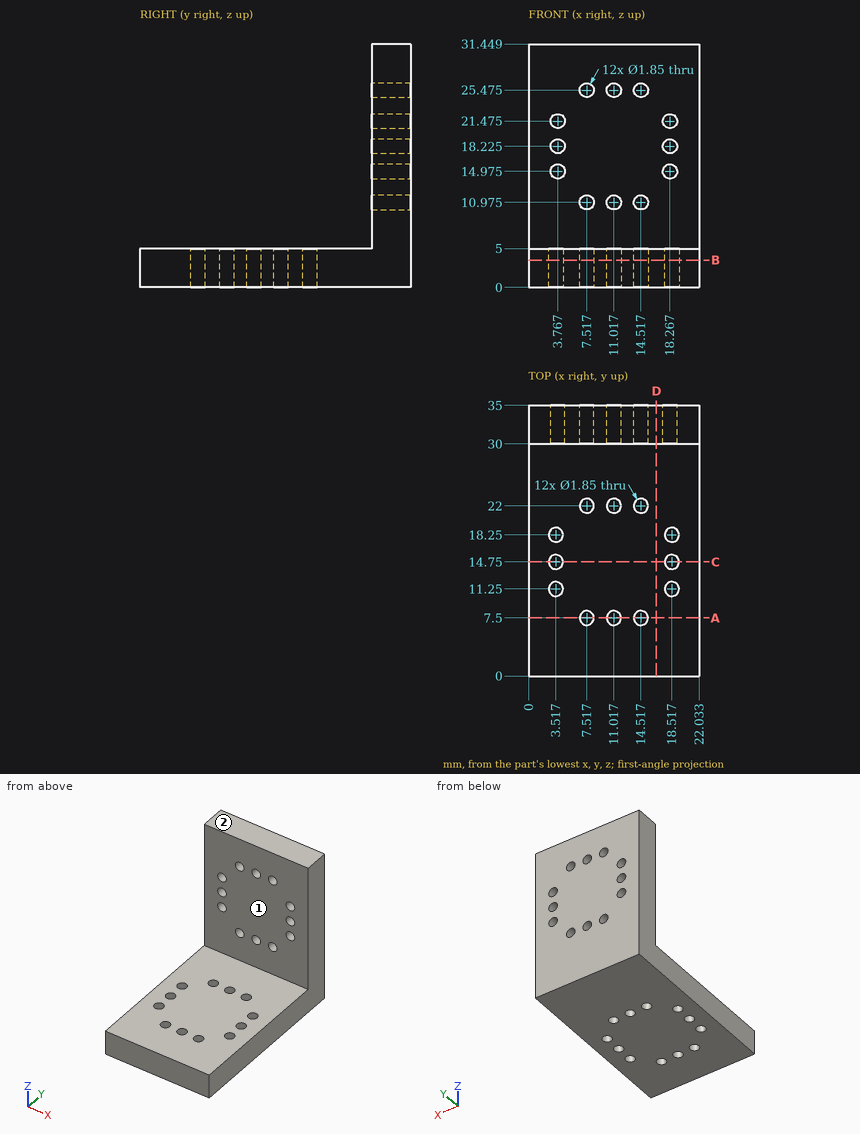
Verification items for this drawing (mm, ordinates from the low corner). A direction names the side the tool comes from. Give positions to 0.01 mm unless a question says otherwise; leave off trailing zeros. Loops run counter-clockwise (first coordinate to the right, second up) from the corner with the lowest first, then second, coordinate; pieces in that order, holes last. Notation, with made-up numbers: M 49.5,36.5 L 98.5,36.5 A35 cw 98.5,74.5 Z; hole C -17.5,54 d7. An arc over 180 degrees is marked long. Answer as CSV lines item,"result".
Item 1: Cross-section at B-B on z = 3.5. Count the separate pieces of the cut face and the enclosed holes in it, and give its area (3 significant figures).
Values:
separate pieces,"1"
enclosed holes,"12"
area,"739 mm²"
Item 2: Cross-section at C-C on y = 14.75. Record the cut outline in (x, z).
Values:
outline,"M 0,0 L 2.59,0 L 2.59,5 L 0,5 Z; M 4.44,0 L 17.59,0 L 17.59,5 L 4.44,5 Z; M 19.44,0 L 22.03,0 L 22.03,5 L 19.44,5 Z"
Item 3: Cross-section at A-A on y = 7.5. Record the cut outline in (x, z).
Values:
outline,"M 0,0 L 6.59,0 L 6.59,5 L 0,5 Z; M 8.44,0 L 10.09,0 L 10.09,5 L 8.44,5 Z; M 11.94,0 L 13.59,0 L 13.59,5 L 11.94,5 Z; M 15.44,0 L 22.03,0 L 22.03,5 L 15.44,5 Z"
Item 4: Access from +Z, -Z, +X, -X, +Y, -Y to the whole of each face (thin tool, end or side, straight path). Record for the marked faces 1 and 2.
Values:
face 1,"+Z, +X, -X, -Y"
face 2,"+Z, +X, -X, +Y, -Y"
Item 5: Material ranges on line 1 (X direction, y = 18.25, z = 1); line 2 (X direction, y = 22, z = 1.5); line 3 (Y direction, x = 17.25, z = 10.5), recorded low to high.
Values:
line 1,"x = 0 to 2.59, 4.44 to 17.59, 19.44 to 22.03"
line 2,"x = 0 to 6.59, 8.44 to 10.09, 11.94 to 13.59, 15.44 to 22.03"
line 3,"y = 30 to 35"
Item 6: Depth check by flat-ended pin: P1, Ø1.1, axis at x = 14.52, z = 10.97, coming from the -Y side; P2, Ø1, axis at x = 4.5, y = 4.5, coming from the +Z side; P3, Ø2.5, axis at x = 11.02, y = 7.5, coming from the -Z side. Enter the tip coordinate at first touch or a pass-through.
Values:
P1,"passes through"
P2,"stops at z = 5"
P3,"stops at z = 0"
Item 7: Cross-section at D-D on x = 16.5. Record the cut outline in (y, z).
Values:
outline,"M 0,0 L 35,0 L 35,31.45 L 30,31.45 L 30,5 L 0,5 Z"
